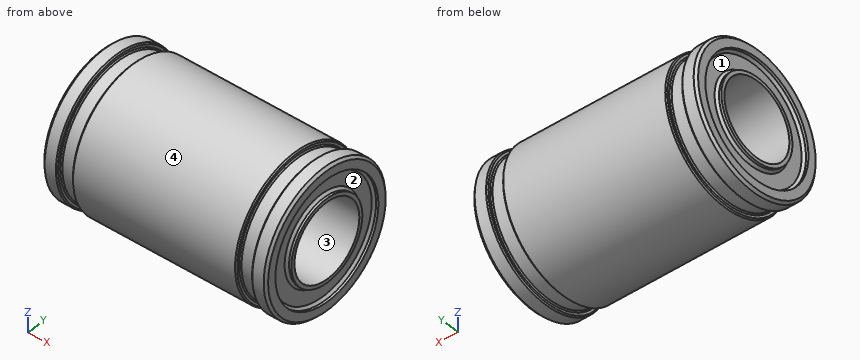
Autodesk Inventor part; units mm, degrees
ref_plane "YZ Plane" through (0, 0, 0) normal (1, 0, 0) x (0, 1, 0)
ref_plane "XZ Plane" through (0, 0, 0) normal (0, 1, 0) x (-1, 0, 0)
ref_plane "XY Plane" through (0, 0, 0) normal (0, 0, 1) x (1, 0, 0)
sketch "Sketch1" plane through (0, 0, 0) normal (0, 0, 1) x (1, 0, 0)
  line L0 (0, 0) -> (23.5, 0)
  line L1 (0, 0) -> (0, 4) construction
  line L2 (0, 4) -> (23.5, 4) construction
  line L3 (0, 0) -> (0, 7.5) construction
  line L4 (0, 7.5) -> (23.5, 7.5) construction
  line L5 (23.5, 7.5) -> (23.5, 0) construction
  line L6 (0, 7.5) -> (23.5, 7.5)
  line L7 (1.5875, 7.5) -> (1.5875, 6.992)
  line L8 (1.5875, 6.992) -> (3.175, 6.992)
  line L9 (3.175, 6.992) -> (3.175, 7.5)
  line L10 (0, 7.5) -> (24, 7.5)
  line L11 (0, 4) -> (24, 4)
  line L12 (24, 4) -> (24, 4.3755)
  line L13 (24, 4.3755) -> (23.5, 4.3755)
  line L14 (23.5, 6.35) -> (24, 6.35)
  line L15 (24, 6.35) -> (24, 7.5)
  line L16 (0, 7.5) -> (0, 6.35)
  line L17 (0, 4) -> (0, 4.3755)
  line L18 (0.5103, 4.3755) -> (0, 4.3755)
  line L19 (0.5103, 4.3755) -> (0.5103, 6.35)
  line L20 (0.5103, 6.35) -> (0, 6.35)
  line L21 (24, 7.5) -> (22.3998, 7.5)
  line L22 (22.3998, 7.5) -> (22.3998, 6.992)
  line L23 (22.3998, 6.992) -> (20.7996, 6.992)
  line L24 (20.7996, 6.992) -> (20.7996, 7.5)
  line L25 (0, 7.5) -> (0, 6.35)
  line L26 (0, 6.35) -> (0.5103, 6.35)
  line L27 (0.5103, 6.35) -> (0.5103, 4.3755)
  line L28 (0, 4) -> (24, 4)
  line L29 (23.5, 6.35) -> (23.5, 4.3755)
  line L30 (22.3998, 7.5) -> (24, 7.5)
  line L31 (24, 7.5) -> (24, 6.35)
  line L32 (22.3998, 7.5) -> (22.3998, 6.992)
  line L33 (22.3998, 6.992) -> (20.7996, 6.992)
  line L34 (20.7996, 6.992) -> (20.7996, 7.5)
  dimension "d0" = 23.5
  dimension "d1" = 4
  dimension "d2" = 7.5
  dimension "d3" = 0.508
  dimension "d4" = 24
  dimension "d5" = 24
  dimension "d6" = 1.6002
  dimension "d7" = 1.6002
revolve "Revolution1" add sketch "Sketch1" angle 360 about axis through (0, 0, 0) along (1, 0, 0) contours L6 L7 L8 L9 L24 L23 L22 L10 L15 L14 L29 L13 L12 L11 L17 L18 L19 L20 L16
chamfer "Chamfer1" distance 0.254 angle 45 6 edges at (24, -7.5, 0) (0, -7.5, 0) (23.5, -4.3755, 0) (23.5, -6.35, 0) (0.5103, -6.35, 0) (0.5103, -4.3755, 0)
chamfer "Chamfer2" distance 0.127 angle 45 8 edges at (3.175, -7.5, 0) (3.175, -6.992, 0) (22.3998, -7.5, 0) (22.3998, -6.992, 0) (1.5875, -6.992, 0) (20.7996, -6.992, 0) (20.7996, -7.5, 0) (1.5875, -7.5, 0)
properties part number "LM8UU 8mm Linear Bearing"
CAD build for the part. Positions are in the model's coordinates, mm. Face numbers are marked on the shaded views. A direction names the side the tool comes from. Round coordinates to 2 decimals unless told otherwise and drop trailing zeros. Write each loop counter-clockwise with the first axis right and the second up, starting at its lowest first coordinate (ties: lowest second). Pieces come first, ordered by that corner, then holes.
(1) Mould opens along Y. For the marked faces 3 and 4 say: pulls with the +Y half, pulls with the -Y half, needs draft (parallel to the pull), parting line crosses it, or undercut.
(2) Slice it at B-B, the plane x = 22. Write the cut outline in (y, z), and give its area (3 significant figures).
(3) Probe line 1 along Z through (x, y) = (23.95, 0); line 2 along X through (y, z) = (5.25, -4.75); line 3 along X through (y, z) = (-6.5, -3) (1 decimal). List the from-to ranges inside material, lowest first.
(4) Drop flat-ended pins along their axis: P1, Ø4, axis at x = 19, z = -5.5, coming from the -Y side; P2, Ø5, axis at x = 19.5, z = 3.5, coming from the -Y side; P3, Ø8, axis at x = 17, y = -6, coming from the -Z side. Give the stop position or say it passes through.
(5) Slice it at A-A, the plane x = 17. Write the cut outline in (y, z).
(6) 3-axis set-ups, long thin cutter, end or side, ignore diameter. For the marked faces 1 and 2: which of +Z, -Z, +X, -X, +Y, -Y reach the whole face in a straight line?
From the geometry:
1. face 3: undercut
1. face 4: parting line crosses it
2. outline: circle Ø13.98 at (0, 0); hole circle Ø8 at (0, 0)
2. area: 103 mm2
3. line 1: z = -7.3 to -6.35, -4.38 to -4, 4 to 4.38, 6.35 to 7.3
3. line 2: x = 0 to 1.63, 3.14 to 20.84, 22.36 to 24
3. line 3: x = 0 to 1.6, 3.2 to 20.8, 22.4 to 24
4. P1: stops at y = -6.63
4. P2: stops at y = -7.43
4. P3: stops at z = -7.23
5. outline: circle Ø15 at (0, 0); hole circle Ø8 at (0, 0)
6. face 1: -X
6. face 2: +X
